Part model, mm, in its own coordinate system. A direction names the side the tool comes from. Round coordinates to 2 decimals unless told otherwise and drop trailing zeros. Loops run counter-clockwise (first coordinate to the right, second up) from the corner with the lowest first, then second, coordinate; pieces in that order, holes last. Notation, with made-up numbers: (-27.5, 62) - (-21.5, 62) arc R9 cw to (-21.5, 70) - close; hole circle Ø10 at (15.25, 84.5). An arc over 180 degrees is marked (long way). Write each question's results on one line, items separated by ' | '. Start each with the question number.
(1) Cut at A-A, the plane x = 0. List the corners of the cut face in (y, z).
(2) Flat gauge pins, fed straight in: P1, Ø3, axis at x = 18, z = -15.5, coming from the -Y side; P2, Ø1, axis at x = -4.5, y = -37, coming from the +Z side; P3, Ø4, axis at y = -28.5, z = 2, coming from the -X side. Where does each tip first touch, or does it go through?
(3) Drill centre lines: L1, parallel to Y at x = 1.5, z = -15; L2, parallel to Y at x = -1.5, z = 3.5; L3, parallel to X at y = -30.5, z = -0.5. Where is each one in solid material? Low to high.
(4) Cut at D-D, the plane z = 15. List the corners of the cut face in (x, y), then the cut area to 3 significant figures.
(5) Cut at C-C, the plane z = 0. List the corners of the cut face in (x, y).
(6) Cut at B-B, the plane y = -26.5. List the corners of the cut face in (x, z), then the cut area to 3 significant figures.
(7) Tool access for faces 1 (the face through (-2.73, -32.34, -12.28)), 2 (the face through (-0.18, -38.21, -0.18)): list every direction of +Z, -Z, +X, -X, +Y, -Y with a clear straight run to the whole face (end or side of a thin tool).
from build123d import *

# Parameters (mm, degrees)
F0_W          = 65.6240805984
F0_H          = 51.0048568249
F1_DEPTH      = 25.4
F2_R          = 12.5804275278
F3_DEPTH      = 25.4
F5_DEPTH      = 25.4
F5_DEPTH_BACK = 25.4


with BuildPart() as f1:
    # F0 (on Front) → F1 (new body)
    with BuildSketch(Plane.XZ):
        Rectangle(F0_W, F0_H)
    extrude(amount=F1_DEPTH)

    # F2 (on face) → F3 (join)
    with BuildSketch(Plane.XZ.offset(25.4)):
        Circle(F2_R)
    extrude(amount=F3_DEPTH)

    # F4 (on Right) → F5 (cut, two sides)
    with BuildSketch(Plane.YZ) as f5_sk:
        Polygon((-51.2365475297, -13.4750008583), (-43.6296612024, -12.7267818898), (-32.5310863554, 12.9620563239), (-51.2365475297, 12.9620563239), align=None)
    extrude(amount=-F5_DEPTH, mode=Mode.SUBTRACT)
    extrude(f5_sk.sketch, amount=F5_DEPTH_BACK, mode=Mode.SUBTRACT)


solid = f1.part
A:
1) outline: (-43.57, -12.58) - (-25.4, -12.58) - (-25.4, -25.5) - (0, -25.5) - (0, 25.5) - (-25.4, 25.5) - (-25.4, 12.58) - (-32.7, 12.58) - close
2) P1: y = -25.4 | P2: z = 3.78 | P3: x = -12.58
3) L1: -25.4 to 0 | L2: -36.62 to 0 | L3: -12.57 to 12.57
4) outline: (-32.81, -25.4) - (32.81, -25.4) - (32.81, 0) - (-32.81, 0) - close | area: 1,670 mm2
5) outline: (-32.81, -25.4) - (-12.58, -25.4) - (-12.58, -38.13) - (12.58, -38.13) - (12.58, -25.4) - (32.81, -25.4) - (32.81, 0) - (-32.81, 0) - close
6) outline: circle Ø25.16 at (0, 0) | area: 497 mm2
7) face 1: -Y | face 2: +Z, +X, -X, -Y
